Part model, mm, in its own coordinate system. Face numbers are marked on the shaded views. A direction names the side the tool comes from. Round coordinates to 2 decimals unless told otherwise and drop trailing zeros. Order: outer loops, then holes, each group sorted by start corner. A loop starts at its lowest first (then second) coordinate and runs counter-clockwise, first axis right, second up. Notation, with made-up numbers: (60.5, -5.75) - (110.5, -5.75) arc R33 cw to (110.5, 24.25) - close; hole circle Ø6 at (84.25, 44.5). An arc over 180 degrees is marked (long way). Return JSON: item names as keys, results as strings. Group by question number.
Item 1: Drop flat-ended pins along their axis: pin 1 (2 mm diameter, centred on x = 31.5, z = 2, fed in from +Y); pin 2 (1.2 mm diameter, centred on x = 36, z = 2.5, fed in from +Y); pin 3 (6 mm diameter, centred on x = 15, y = 0, fed in from +Z); pin 4 (4 mm diameter, centred on x = 0, y = 0, fed in from -Z). Give the stop position or say it passes through.
Item 2: Two-plate mould, pull along Y, no slides. Class the marked faces 1, 2 and 3: released by +Y, released by -Y, zero draft, split by the parting line, or undercut.
Item 3: Tool access for the marked faces 4, 5, 6, 7 and 8: list every direction of +Z, -Z, +X, -X, +Y, -Y with a clear straight run to the whole face (end or side of a thin tool).
Item 4: Probe probe 1 along Y at (x, z) = (0, 0.45); probe 2 along Y at (x, z) = (39.5, 4.5); probe 3 along X at (y, z) = (0, 0.7). List the from-to ranges inside material, lowest first.
Item 5: Saw through at C-C on x = 0. List the corners of the cut face in (y, z), and give its area (3 significant figures).
Item 6: Saw through at B-B on x = 45.5. List the corners of the cut face in (y, z).
Item 7: Saw through at A-A on y = 0. State how many separate pieces and enclosed holes the cut face has, and give its area (3 significant figures).
```python
from build123d import *

# Parameters (mm, degrees)
ESQUISSE1_R                  = 3.5
ESQUISSE1_R_2                = 1.5
BOSS_EXTRU_1_DEPTH           = 5
ENL_V_MAT_EXTRU_2_DEPTH      = 50.256979201
ENL_V_MAT_EXTRU_2_DEPTH_BACK = 50.256979201
ENL_V_MAT_EXTRU_3_DEPTH      = 50.580742257
ENL_V_MAT_EXTRU_3_DEPTH_BACK = 50.580742257


with BuildPart() as part:
    # Esquisse1 → Boss.-Extru.1 (new body)
    # profile 1 of 2: a face of its own
    with BuildSketch(Plane.XY):
        Circle(ESQUISSE1_R)
        Circle(ESQUISSE1_R_2, mode=Mode.SUBTRACT)
    # profile 2 of 2: a face of its own
    with BuildSketch(Plane.XY):
        with BuildLine():
            Line((33.05, 2.5), (3.5, 2.5))
            Line((3.5, 2.5), (2.449489743, 2.5))
            ThreePointArc((2.449489743, 2.5), (3.226702194, 1.355873501), (3.5, 0))
            ThreePointArc((3.5, 0), (3.226702194, -1.355873501), (2.449489743, -2.5))
            Line((2.449489743, -2.5), (3.5, -2.5))
            Line((3.5, -2.5), (33.05, -2.5))
            ThreePointArc((33.05, -2.5), (34.428858223, -3.071141777), (35, -4.45))
            Line((35, -4.45), (35, -4.5))
            Line((35, -4.5), (47, -4.5))
            ThreePointArc((47, -4.5), (48.060660172, -4.060660172), (48.5, -3))
            Line((48.5, -3), (48.5, 3))
            ThreePointArc((48.5, 3), (48.060660172, 4.060660172), (47, 4.5))
            Line((47, 4.5), (43.75, 4.5))
            ThreePointArc((43.75, 4.5), (43.219669914, 4.719669914), (43, 5.25))
            Line((43, 5.25), (43, 5.5))
            Line((43, 5.5), (40.5, 5.5))
            Line((40.5, 5.5), (40.5, 5.25))
            ThreePointArc((40.5, 5.25), (40.280330086, 4.719669914), (39.75, 4.5))
            Line((39.75, 4.5), (35, 4.5))
            Line((35, 4.5), (35, 4.45))
            ThreePointArc((35, 4.45), (34.428858223, 3.071141777), (33.05, 2.5))
        make_face()
        Polygon((41.5, -3), (37, -3), (37, 3), (41.5, 3), (41.5, 2.5), (46.5, 2.5), (46.5, -2.5), (41.5, -2.5), align=None, mode=Mode.SUBTRACT)
    extrude(amount=BOSS_EXTRU_1_DEPTH)

    # Esquisse2 → Enlèv. mat.-Extru.2 (cut, two sides: drawn at the far end of the back side and taken through both)
    with BuildSketch(Plane(origin=(0, 2.5, 0), x_dir=(1, 0, 0), z_dir=(0, 1, 0)).offset(-ENL_V_MAT_EXTRU_2_DEPTH_BACK)):
        with BuildLine():
            ThreePointArc((5.449489743, -0.5), (5.595936352, -0.853553391), (5.949489743, -1))
            Line((5.949489743, -1), (48.5, -1))
            Line((48.5, -1), (48.5, 0))
            Line((48.5, 0), (5.049489743, 0))
            ThreePointArc((5.049489743, 0), (5.332332455, -0.117157288), (5.449489743, -0.4))
            Line((5.449489743, -0.4), (5.449489743, -0.5))
        make_face()
        with BuildLine():
            Line((4.849489662, -5), (35.098076211, -5))
            ThreePointArc((35.098076211, -5), (34, -3.901923789), (32.5, -3.5))
            Line((32.5, -3.5), (6.249489662, -3.5))
            ThreePointArc((6.249489662, -3.5), (5.683804237, -3.734314575), (5.449489662, -4.3))
            Line((5.449489662, -4.3), (5.449489662, -4.4))
            ThreePointArc((5.449489662, -4.4), (5.27375373, -4.824264069), (4.849489662, -5))
        make_face()
        with BuildLine():
            Line((4.295064523, -1.5), (-3.5, -1.5))
            Line((-3.5, -1.5), (-3.5, -3.5))
            Line((-3.5, -3.5), (4.295064523, -3.5))
            ThreePointArc((4.295064523, -3.5), (5.295064523, -2.5), (4.295064523, -1.5))
        make_face()
    extrude(amount=ENL_V_MAT_EXTRU_2_DEPTH + ENL_V_MAT_EXTRU_2_DEPTH_BACK, mode=Mode.SUBTRACT)

    # Esquisse3 → Enlèv. mat.-Extru.3 (cut, two sides: drawn at the far end of the back side and taken through both)
    with BuildSketch(Plane(origin=(0, 4.5, 0), x_dir=(1, 0, 0), z_dir=(0, 1, 0)).offset(-ENL_V_MAT_EXTRU_3_DEPTH_BACK)):
        with BuildLine():
            Line((37.750303976, -4), (37.250303976, -4))
            ThreePointArc((37.250303976, -4), (36.250303976, -3), (37.250303976, -2))
            Line((37.250303976, -2), (37.750303976, -2))
            ThreePointArc((37.750303976, -2), (38.750303976, -3), (37.750303976, -4))
        make_face()
    extrude(amount=ENL_V_MAT_EXTRU_3_DEPTH + ENL_V_MAT_EXTRU_3_DEPTH_BACK, mode=Mode.SUBTRACT)


solid = part.part
```
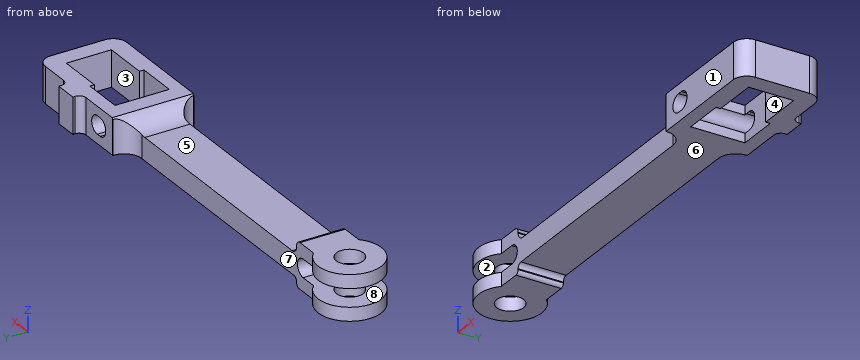
Filled in:
{
 "1": {"pin 1": "stops at y = 2.5", "pin 2": "stops at y = 4.5", "pin 3": "stops at z = 3.5", "pin 4": "stops at z = 0"},
 "2": {"face 1": "released by -Y", "face 2": "zero draft", "face 3": "undercut"},
 "3": {"face 4": "+Z, -Z", "face 5": "+Z, +Y, -Y", "face 6": "-Z, +X, +Y, -Y", "face 7": "+Z, -Z, +Y", "face 8": "-X, +Y, -Y"},
 "4": {"probe 1": "y = -3.5 to -1.5, 1.5 to 3.5", "probe 2": "y = -4.5 to -3, 3 to 4.5", "probe 3": "x = -3.5 to -1.5, 1.5 to 5.49"},
 "5": {"outline": "(-3.5, 0) - (-1.5, 0) - (-1.5, 1.5) - (-3.5, 1.5) - close; (-3.5, 3.5) - (-1.5, 3.5) - (-1.5, 5) - (-3.5, 5) - close; (1.5, 0) - (3.5, 0) - (3.5, 1.5) - (1.5, 1.5) - close; (1.5, 3.5) - (3.5, 3.5) - (3.5, 5) - (1.5, 5) - close", "area": "12.0 mm^2"},
 "6": {"outline": "(-4.5, 1) - (-2.5, 1) - (-2.5, 5) - (-4.5, 5) - close; (2.5, 1) - (4.5, 1) - (4.5, 5) - (2.5, 5) - close"},
 "7": {"separate pieces": "4", "enclosed holes": "0", "area": "108 mm^2"}
}
